Read the model definition and answer for the solid it produces. Units are mm, in the model's axes. A direction names the side the tool comes from. Coordinates: 2 decimals unless noted, no trailing zeros. Order: outer loops, then holes, each group sorted by start corner. A loop starts at its lowest first (then second) coordinate and runs counter-clockwise, first axis right, second up. Notation, with made-up numbers: (29, 28.5) - (53, 28.5) arc R7 ccw to (53, 36.5) - close; hole circle Ø9 at (9, 59.25). An arc over 180 degrees is marked (long way). Use one line per item in the form item = value.
```python
from build123d import *

# Parameters (mm, degrees)
F0_W      = 100
F0_H      = 54
F1_DEPTH  = 1.45
F2_W      = 87
F2_H      = 50.3
F3_DEPTH  = 10.1
F4_R      = 1.25
F5_DEPTH  = 1.451
F7_R      = 0.5
F6_W      = 71.8
F6_H      = 40
F8_DEPTH  = 0.75
F9_R      = 0.5
F10_DEPTH = 1.451


with BuildPart() as f1:
    # F0 (on Top) → F1 (new body)
    with BuildSketch(Plane.XY):
        with Locations((50, 27)):
            Rectangle(F0_W, F0_H)
    extrude(amount=F1_DEPTH)

    # F2 (on face) → F3 (join)
    with BuildSketch(Plane.XY.offset(1.45)):
        with Locations((51.2, 28.85)):
            Rectangle(F2_W, F2_H)
    extrude(amount=F3_DEPTH)

    # F4 (on face) → F5 (cut, through all)
    with BuildSketch(Plane.XY.offset(1.45)):
        with Locations((2.5, 51.5)):
            Circle(F4_R)
        with Locations((2.5, 2.5)):
            Circle(F4_R)
        with Locations((97.5, 2.5)):
            Circle(F4_R)
        with Locations((97.5, 51.5)):
            Circle(F4_R)
    extrude(amount=-F5_DEPTH, mode=Mode.SUBTRACT)

    # F7
    f7_edges = [f1.edges().sort_by_distance(p)[0] for p in [
        (7.7, 28.85, 11.55),
        (51.2, 54, 11.55),
        (51.2, 3.7, 11.55),
        (94.7, 28.85, 11.55),
    ]]
    fillet(f7_edges, radius=F7_R)

    # F6 (on face) → F8 (cut)
    with BuildSketch(Plane.XY.offset(11.55)):
        with Locations((51.2, 28.8)):
            Rectangle(F6_W, F6_H)
    extrude(amount=-F8_DEPTH, mode=Mode.SUBTRACT)

    # F9 (on face) → F10 (cut, through all)
    with BuildSketch(Plane.XY.offset(1.45)):
        with Locations((90, 1.6)):
            Circle(F9_R)
        with Locations((87.46, 1.6)):
            Circle(F9_R)
        with Locations((84.92, 1.6)):
            Circle(F9_R)
        with Locations((82.38, 1.6)):
            Circle(F9_R)
        with Locations((79.84, 1.6)):
            Circle(F9_R)
        with Locations((77.3, 1.6)):
            Circle(F9_R)
        with Locations((74.76, 1.6)):
            Circle(F9_R)
        with Locations((72.22, 1.6)):
            Circle(F9_R)
        with Locations((69.68, 1.6)):
            Circle(F9_R)
        with Locations((67.14, 1.6)):
            Circle(F9_R)
        with Locations((64.6, 1.6)):
            Circle(F9_R)
        with Locations((62.06, 1.6)):
            Circle(F9_R)
        with Locations((59.52, 1.6)):
            Circle(F9_R)
        with Locations((56.98, 1.6)):
            Circle(F9_R)
        with Locations((54.44, 1.6)):
            Circle(F9_R)
        with Locations((51.9, 1.6)):
            Circle(F9_R)
        with Locations((49.36, 1.6)):
            Circle(F9_R)
        with Locations((46.82, 1.6)):
            Circle(F9_R)
        with Locations((44.28, 1.6)):
            Circle(F9_R)
        with Locations((41.74, 1.6)):
            Circle(F9_R)
    extrude(amount=-F10_DEPTH, mode=Mode.SUBTRACT)


solid = f1.part
```
(1) Which of the six approach directions +Z, -Z, +X, -X, +Y, -Y give full straight-line access (tool end or side, diameter ignored) to faces 1 (the flat face through (7.7, 28, 6)), 2 (the flat face through (51, 3.7, 6)), 3 (the flat face through (49, 27, 0)), 4 (the flat face through (51, 29, 10.8))?
Answer list:
face_1 = +Z, -X, +Y, -Y
face_2 = +Z, +X, -X, -Y
face_3 = -Z, +X, -X, +Y, -Y
face_4 = +Z
(2) Straight lines are drawn through the part: L1, parallel to Y at x = 2.5, z = 0.9; L2, parallel to Y at x = 49.36, z = 1; L3, parallel to Y at x = 40.5, z = 11. For each, find the intervals that lie inside material, in ascending order.
Answer list:
L1 = 0 to 1.25, 3.75 to 50.25, 52.75 to 54
L2 = 0 to 1.1, 2.1 to 54
L3 = 3.7 to 8.8, 48.8 to 54
(3) Section B-B, the plane y = 40.5 is taken. Write down the section's boundary in (x, z), then the cut area to 3 significant figures.
Answer list:
outline = (0, 0) - (100, 0) - (100, 1.45) - (94.7, 1.45) - (94.7, 11.05) arc R0.5 ccw to (94.2, 11.55) - (87.1, 11.55) - (87.1, 10.8) - (15.3, 10.8) - (15.3, 11.55) - (8.2, 11.55) arc R0.5 ccw to (7.7, 11.05) - (7.7, 1.45) - (0, 1.45) - close
area = 970 mm2
(4) Given pin 1 Ø3 at (x, z) = (88.5, 5.5) entering from -Y; pin 2 Ø0.8 at (x, z) = (33.5, 11.5) entering from +Y; pin 3 Ø5 at (x, y) = (83, 24) entering from +Z, each flat-ended and moving along its own axis, determine where each tip first touches the part or whether it passes through.
Answer list:
pin_1 = 3.7
pin_2 = 54
pin_3 = 10.8
(5) Section A-A, the plane x = 97.5 is taken. Write down the section's boundary in (y, z), then the cut area to 4 significant figures.
Answer list:
outline = (0, 0) - (1.25, 0) - (1.25, 1.45) - (0, 1.45) - close; (3.75, 0) - (50.25, 0) - (50.25, 1.45) - (3.75, 1.45) - close; (52.75, 0) - (54, 0) - (54, 1.45) - (52.75, 1.45) - close
area = 71.05 mm2
(6) Section C-C, the plane z = 5 is taken. Write down the section's boundary in (x, y), then the cut area to 3 significant figures.
Answer list:
outline = (7.7, 3.7) - (94.7, 3.7) - (94.7, 54) - (7.7, 54) - close
area = 4,380 mm2
(7) The mould has two halves that part along Y. Classify faces 5 (the flat face through (94.7, 28, 6)), 6 (the flat face through (49, 54, 5)), 7 (the cylindrical face through (3.69, 2.88, 0.74)): +Y half, -Y half, draft (parallel to the pull), parting line (faces both ways), or undercut.
Answer list:
face_5 = draft
face_6 = +Y half
face_7 = undercut
